Check sheet for the modelled part. Datum: model origin and axes. Units: mm. Give positions to 0.01 mm unless a question says otherwise; leave off trailing zeros. Loops run counter-clockwise (first coordinate to the right, second up) from the corner with the lowest first, then second, coordinate; pieces in that order, holes last. Notation, with made-up numbers: M 30.25,14 L 83.25,14 A34 cw 83.25,47 Z; hole C 23.5,-34.5 d8. An arc over 180 degrees is marked long. Write each question's results on one line, items separated by ' | '. Start each with the question number.
1. Material ranges on line 1 along X through (y, z) = (25, 2.25); line 2 along Y through (x, z) = (24, 0.2); line 3 along Y through (x, z) = (-21, 1.4), recorded low to high.
2. Sectioned sample at A-A on x = -10.5. Record the cut outline in (y, z).
3. Sectioned sample at B-B on x = 32. Record the cut outline in (y, z), and give its area (3 significant figures).
4. Go/stop test with flat-tipped pins: pin 1 (1.2 mm diameter, centred on y = 24, z = 2, fed in from -X); pin 2 (2.5 mm diameter, centred on y = -24, z = 2, fed in from -X); pin 3 (1.4 mm diameter, centred on x = -24.5, y = 7.5, fed in from +Z). Record where each tip stops, or that it passes through.
5. Draft check along Y on faces 1 (the cylindrical face through (-8.67, -39.05, 0.96)), 2 (the flat face through (-2, 24, 2)). Enter one of: pulls with the +Y half, pulls with the -Y half, needs draft (parallel to the pull), parting line crosses it, or undercut.
6. Sectioned sample at C-C on y = 31.5. Record the cut outline in (x, z).
```python
from build123d import *

# Parameters (mm, degrees)
SKETCH2_R           = 40
SKETCH2_R_2         = 2
SKETCH2_R_3         = 1
BOSS_EXTRUDE1_DEPTH = 4
SKETCH2_3_R         = 2
SKETCH2_3_R_2       = 1
CUT_EXTRUDE2_DEPTH  = 10
CIRPATTERN1_COUNT   = 10
BOSS_EXTRUDE2_START = -2
SKETCH2_4_R         = 40
SKETCH2_4_R_2       = 2
SKETCH2_4_R_3       = 1
BOSS_EXTRUDE2_DEPTH = 2


with BuildPart() as part:
    # Sketch2 → Boss-Extrude1 (new body)
    # profile 1 of 6: a face of its own
    with BuildSketch(Plane.XY):
        Circle(SKETCH2_R)
        with BuildLine():
            Line((-9.449023862, 21.516643513), (-9.449023862, 25.845037204))
            Line((-9.449023862, 25.845037204), (-7.546910829, 26.463071192))
            Line((-7.546910829, 26.463071192), (-5.002744851, 22.961327138))
            ThreePointArc((-5.002744851, 22.961327138), (-3.508704096, 23.236587434), (-2, 23.414738948))
            Line((-2, 23.414738948), (-2, 25.5))
            ThreePointArc((-2, 25.5), (0, 27.5), (2, 25.5))
            Line((2, 25.5), (2, 23.414738948))
            ThreePointArc((2, 23.414738948), (17.309679373, 15.894181325), (23.5, 0))
            ThreePointArc((23.5, 0), (-12.849084389, -19.676153851), (-9.449023862, 21.516643513))
        make_face(mode=Mode.SUBTRACT)
    # profile 2 of 6: a face of its own
    with BuildSketch(Plane.XY):
        with BuildLine():
            Line((-7.546910829, 26.463071192), (-9.449023862, 25.845037204))
            Line((-9.449023862, 25.845037204), (-9.449023862, 21.516643513))
            ThreePointArc((-9.449023862, 21.516643513), (-7.261899368, 22.349828133), (-5.002744851, 22.961327138))
            Line((-5.002744851, 22.961327138), (-7.546910829, 26.463071192))
        make_face()
    # profile 3 of 6: a face of its own
    with BuildSketch(Plane.XY):
        with Locations((0, 25.5)):
            Circle(SKETCH2_R_2)
        with Locations((0, 25.5)):
            Circle(SKETCH2_R_3, mode=Mode.SUBTRACT)
    # profile 4 of 6: a face of its own
    with BuildSketch(Plane.XY):
        with BuildLine():
            Line((-2, 25.5), (-2, 23.414738948))
            ThreePointArc((-2, 23.414738948), (-1.000908268, 23.478675061), (0, 23.5))
            ThreePointArc((0, 23.5), (-1.414213562, 24.085786438), (-2, 25.5))
        make_face()
    # profile 5 of 6: a face of its own
    with BuildSketch(Plane.XY):
        with Locations((0, 25.5)):
            Circle(SKETCH2_R_3)
    # profile 6 of 6: a face of its own
    with BuildSketch(Plane.XY):
        with BuildLine():
            ThreePointArc((0, 23.5), (1.000908268, 23.478675061), (2, 23.414738948))
            Line((2, 23.414738948), (2, 25.5))
            ThreePointArc((2, 25.5), (1.414213562, 24.085786438), (0, 23.5))
        make_face()
    extrude(amount=BOSS_EXTRUDE1_DEPTH)

    # Sketch2_3 → Cut-Extrude2 (cut)
    # profile 1 of 5: a face of its own
    with BuildSketch(Plane.XY):
        with BuildLine():
            Line((-7.546910829, 26.463071192), (-9.449023862, 25.845037204))
            Line((-9.449023862, 25.845037204), (-9.449023862, 21.516643513))
            ThreePointArc((-9.449023862, 21.516643513), (-7.261899368, 22.349828133), (-5.002744851, 22.961327138))
            Line((-5.002744851, 22.961327138), (-7.546910829, 26.463071192))
        make_face()
    # profile 2 of 5: a face of its own
    with BuildSketch(Plane.XY):
        with Locations((0, 25.5)):
            Circle(SKETCH2_3_R)
        with Locations((0, 25.5)):
            Circle(SKETCH2_3_R_2, mode=Mode.SUBTRACT)
    # profile 3 of 5: a face of its own
    with BuildSketch(Plane.XY):
        with Locations((0, 25.5)):
            Circle(SKETCH2_3_R_2)
    # profile 4 of 5: a face of its own
    with BuildSketch(Plane.XY):
        with BuildLine():
            Line((-2, 25.5), (-2, 23.414738948))
            ThreePointArc((-2, 23.414738948), (-1.000908268, 23.478675061), (0, 23.5))
            ThreePointArc((0, 23.5), (-1.414213562, 24.085786438), (-2, 25.5))
        make_face()
    # profile 5 of 5: a face of its own
    with BuildSketch(Plane.XY):
        with BuildLine():
            ThreePointArc((0, 23.5), (1.000908268, 23.478675061), (2, 23.414738948))
            Line((2, 23.414738948), (2, 25.5))
            ThreePointArc((2, 25.5), (1.414213562, 24.085786438), (0, 23.5))
        make_face()
    cut_extrude2 = extrude(amount=CUT_EXTRUDE2_DEPTH, mode=Mode.SUBTRACT)

    # CirPattern1: Cut-Extrude2 ×10 about axis
    cirpattern1_axis = Axis((0, 0, 0), (0, 0, 1))
    for i in range(1, CIRPATTERN1_COUNT):
        add(cut_extrude2.rotate(cirpattern1_axis, i * 360 / CIRPATTERN1_COUNT), mode=Mode.SUBTRACT)

    # Sketch2_4 → Boss-Extrude2 (add)
    # profile 1 of 6: a face of its own
    with BuildSketch(Plane.XY.offset(BOSS_EXTRUDE2_START)):
        Circle(SKETCH2_4_R)
        with BuildLine():
            Line((-9.449023862, 21.516643513), (-9.449023862, 25.845037204))
            Line((-9.449023862, 25.845037204), (-7.546910829, 26.463071192))
            Line((-7.546910829, 26.463071192), (-5.002744851, 22.961327138))
            ThreePointArc((-5.002744851, 22.961327138), (-3.508704096, 23.236587434), (-2, 23.414738948))
            Line((-2, 23.414738948), (-2, 25.5))
            ThreePointArc((-2, 25.5), (0, 27.5), (2, 25.5))
            Line((2, 25.5), (2, 23.414738948))
            ThreePointArc((2, 23.414738948), (17.309679373, 15.894181325), (23.5, 0))
            ThreePointArc((23.5, 0), (-12.849084389, -19.676153851), (-9.449023862, 21.516643513))
        make_face(mode=Mode.SUBTRACT)
    # profile 2 of 6: a face of its own
    with BuildSketch(Plane.XY.offset(BOSS_EXTRUDE2_START)):
        with BuildLine():
            ThreePointArc((0, 23.5), (1.000908268, 23.478675061), (2, 23.414738948))
            Line((2, 23.414738948), (2, 25.5))
            ThreePointArc((2, 25.5), (1.414213562, 24.085786438), (0, 23.5))
        make_face()
    # profile 3 of 6: a face of its own
    with BuildSketch(Plane.XY.offset(BOSS_EXTRUDE2_START)):
        with BuildLine():
            Line((-2, 25.5), (-2, 23.414738948))
            ThreePointArc((-2, 23.414738948), (-1.000908268, 23.478675061), (0, 23.5))
            ThreePointArc((0, 23.5), (-1.414213562, 24.085786438), (-2, 25.5))
        make_face()
    # profile 4 of 6: a face of its own
    with BuildSketch(Plane.XY.offset(BOSS_EXTRUDE2_START)):
        with Locations((0, 25.5)):
            Circle(SKETCH2_4_R_2)
        with Locations((0, 25.5)):
            Circle(SKETCH2_4_R_3, mode=Mode.SUBTRACT)
    # profile 5 of 6: a face of its own
    with BuildSketch(Plane.XY.offset(BOSS_EXTRUDE2_START)):
        with Locations((0, 25.5)):
            Circle(SKETCH2_4_R_3)
    # profile 6 of 6: a face of its own
    with BuildSketch(Plane.XY.offset(BOSS_EXTRUDE2_START)):
        with BuildLine():
            Line((-7.546910829, 26.463071192), (-9.449023862, 25.845037204))
            Line((-9.449023862, 25.845037204), (-9.449023862, 21.516643513))
            ThreePointArc((-9.449023862, 21.516643513), (-7.261899368, 22.349828133), (-5.002744851, 22.961327138))
            Line((-5.002744851, 22.961327138), (-7.546910829, 26.463071192))
        make_face()
    extrude(amount=BOSS_EXTRUDE2_DEPTH)


solid = part.part
```
Output values:
1) line 1: -31.22 to -9.45, -6.48 to -2, 2 to 6.48, 9.45 to 31.22 | line 2: -32 to -9.86, -5.7 to -2.14, 2.14 to 5.7, 9.86 to 32 | line 3: -34.04 to -16.76, -12.83 to -10.55, 10.55 to 12.83, 16.76 to 34.04
2) outline: M -38.6,-2 L -21.02,-2 L -21.02,4 L -38.6,4 Z; M 21.02,-2 L 38.6,-2 L 38.6,4 L 21.02,4 Z
3) outline: M -24,-2 L 24,-2 L 24,4 L -24,4 Z | area: 288 mm2
4) pin 1: x = -32.44 | pin 2: x = -32.9 | pin 3: z = 0
5) face 1: parting line crosses it | face 2: undercut
6) outline: M -24.65,-2 L 24.65,-2 L 24.65,4 L -24.65,4 Z
